from build123d import *

# Parameters (mm, degrees)
CUBE003_W     = 60.5
CUBE003_H     = 20
CUBE003_DEPTH = 3
CUBE004_W     = 30
CUBE004_H     = 10
CUBE004_DEPTH = 47.5
CUBE002_W     = 40.9
CUBE002_H     = 20.4
CUBE002_DEPTH = 27.9
CUBE001_W     = 60.5
CUBE001_H     = 24
CUBE001_DEPTH = 2
CUBE_W        = 44.5
CUBE_H        = 24
CUBE_DEPTH    = 27.5


with BuildPart() as cube003:
    # cube003 → cube003 (new body)
    with BuildSketch(Plane(origin=(-30.25, -10, 11.75), x_dir=(1, 0, 0), z_dir=(0, 0, 1))):
        with Locations((30.25, 10)):
            Rectangle(CUBE003_W, CUBE003_H)
    extrude(amount=CUBE003_DEPTH)


with BuildPart() as cube004:
    # cube004 → cube004 (new body)
    with BuildSketch(Plane(origin=(5, -5, -11.95), x_dir=(1, 0, 0), z_dir=(0, 0, 1))):
        with Locations((15, 5)):
            Rectangle(CUBE004_W, CUBE004_H)
    extrude(amount=CUBE004_DEPTH)


with BuildPart() as union001:
    # cube002 → cube002 (new body)
    with BuildSketch(Plane(origin=(-20.45, -10.2, -11.95), x_dir=(1, 0, 0), z_dir=(0, 0, 1))):
        with Locations((20.45, 10.2)):
            Rectangle(CUBE002_W, CUBE002_H)
    extrude(amount=CUBE002_DEPTH)

    # union001: union cube003, cube004
    add(cube003.part)
    add(cube004.part)


with BuildPart() as cube001:
    # cube001 → cube001 (new body)
    with BuildSketch(Plane(origin=(-30.25, -12, 9.75), x_dir=(1, 0, 0), z_dir=(0, 0, 1))):
        with Locations((30.25, 12)):
            Rectangle(CUBE001_W, CUBE001_H)
    extrude(amount=CUBE001_DEPTH)


with BuildPart() as difference:
    # cube → cube (new body)
    with BuildSketch(Plane(origin=(-22.25, -12, -13.75), x_dir=(1, 0, 0), z_dir=(0, 0, 1))):
        with Locations((22.25, 12)):
            Rectangle(CUBE_W, CUBE_H)
    extrude(amount=CUBE_DEPTH)

    # union: union cube001
    add(cube001.part)

    # difference: cut union001
    add(union001.part, mode=Mode.SUBTRACT)


solid = difference.part
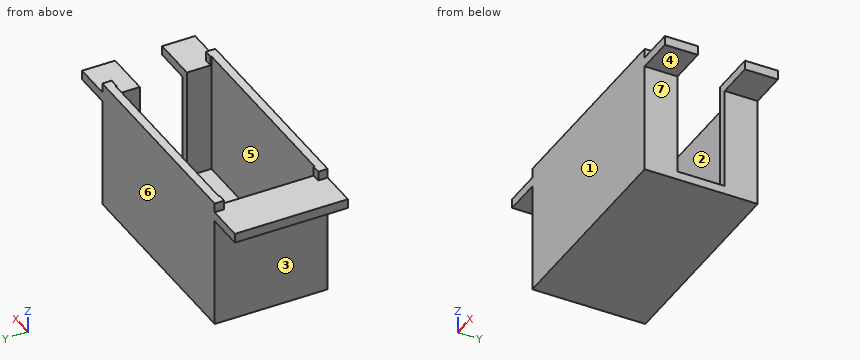
Model file for the job. Use its own axes, mm. Face numbers are marked on the shaded views. A direction names the side the tool comes from. Round coordinates to 2 decimals unless told otherwise and drop trailing zeros. Loops run counter-clockwise (first coordinate to the right, second up) from the corner with the lowest first, then second, coordinate; pieces in that order, holes last.
1. Band-saw the part on C-C, the plane z = -10. List the corners of the cut face in (x, y).
Check values:
outline: (-22.25, -12) - (22.25, -12) - (22.25, -5) - (20.45, -5) - (20.45, -10.2) - (-20.45, -10.2) - (-20.45, 10.2) - (20.45, 10.2) - (20.45, 5) - (22.25, 5) - (22.25, 12) - (-22.25, 12) - close
2. Wall check: probe 1 along X at (y, z) = (-7.5, -9); probe 2 along Y at (x, z) = (17, -10.75); probe 3 along Z at (x, y) = (12, 3.75). Give the ranges that are in metal, low to high.
Check values:
probe 1: x = -22.25 to -20.45, 20.45 to 22.25
probe 2: y = -12 to -10.2, 10.2 to 12
probe 3: z = -13.75 to -11.95
3. Band-saw the part on D-D, the plane y = -6.5. List the corners of the cut face in (x, z).
Check values:
outline: (-30.25, 9.75) - (-22.25, 9.75) - (-22.25, -13.75) - (22.25, -13.75) - (22.25, 9.75) - (30.25, 9.75) - (30.25, 11.75) - (20.45, 11.75) - (20.45, -11.95) - (-20.45, -11.95) - (-20.45, 11.75) - (-30.25, 11.75) - close
4. Drop flat-ended pins along their axis: P1, Ø8, axis at x = -25.5, y = 0.5, coming from the +Z side; P2, Ø4, axis at y = 0.5, z = -6, coming from the +X side; P3, Ø1, axis at y = 11, z = 13, coming from the -X side. Give the stop position or say it passes through.
Check values:
P1: stops at z = 11.75
P2: stops at x = -20.45
P3: stops at x = -22.25
5. Band-saw the part on B-B, the plane y = -1.5. List the corners of the cut face in (x, z).
Check values:
outline: (-30.25, 9.75) - (-22.25, 9.75) - (-22.25, -13.75) - (22.25, -13.75) - (22.25, -11.95) - (-20.45, -11.95) - (-20.45, 11.75) - (-30.25, 11.75) - close
6. Mould opens along Y. For the marked faces 5, 6 and 7 say: +Y half, -Y half, draft (parallel to the pull), parting line (faces both ways), or undercut.
Check values:
face 5: undercut
face 6: +Y half
face 7: draft
7. Band-saw the part on A-A, the plane x = 14. List the corners of the cut face in (y, z), and give its area (3 significant figures).
Check values:
outline: (-12, -13.75) - (12, -13.75) - (12, 13.75) - (10.2, 13.75) - (10.2, -11.95) - (-10.2, -11.95) - (-10.2, 13.75) - (-12, 13.75) - close
area: 136 mm2
8. Tool access for the marked faces 1, 2, 3 and 4: list every direction of +Z, -Z, +X, -X, +Y, -Y with a clear straight run to the whole face (end or side of a thin tool).
Check values:
face 1: +Z, -Z, +X, -X, -Y
face 2: +Z
face 3: -Z, -X, +Y, -Y
face 4: -Z, +X, +Y, -Y
